Input: part model. Units: mm. Frame: model coordinates. Coordinates: 2 decimals unless noted, no trailing zeros. Order: outer loops, then holes, each group sorted by start corner. A loop starts at its lowest first (then second) coordinate and runs counter-clockwise, first axis right, second up. Notation, with made-up numbers: (17, 58) - (36, 58) arc R18 ccw to (36, 67) - close; hole circle Ø5 at (56.5, 79.25). An arc over 180 degrees is marked (long way). Answer as CSV lines item,"result". Start each with the question number.
Item 1: Material intervals for line 1 along X through (y, z) = (0.5, -184.5); line 2 along Y through (x, z) = (0, 91); line 3 along Y through (x, z) = (0, 218), sorted ascending.
Item 2: Section C-C (z = -195.5). Output: boundary loops of the cut face in (x, y), and give its area (3 significant figures).
Item 3: First-contact query: pin 1 (2 mm diameter, centred on y = -14, z = 18, fed in from -X); pin 2 (5 mm diameter, centred on y = 8, z = 146.5, fed in from -X); pin 3 (1.5 mm diameter, centred on y = 18.5, z = -55, fed in from -X). Flat tips, straight axial feed; report the tip coordinate or a pass-through.
Item 4: Section A-A (x = 0). Output: boundary loops of the cut face in (y, z).
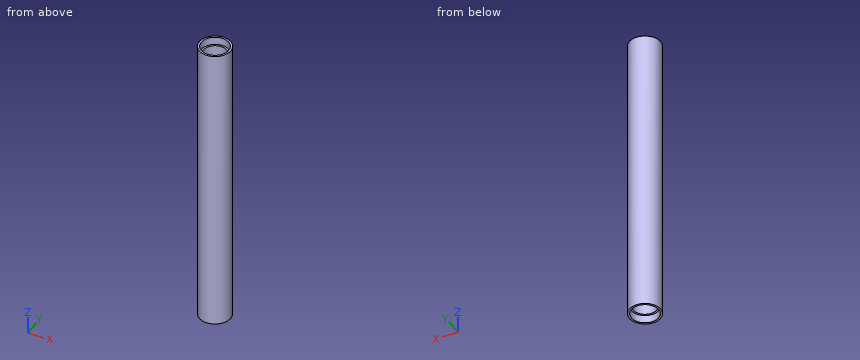
from build123d import *

# Parameters (mm, degrees)
SKETCH_1_R      = 24
SKETCH_1_R_2    = 21
EXTRUDE_1_DEPTH = 225
EXTRUDE_START   = -225
SKETCH_2_R      = 21
SKETCH_2_R_2    = 18
EXTRUDE_2_DEPTH = 213


with BuildPart() as part:
    # 草图1 → 拉伸-薄壁1 (new, symmetric)
    with BuildSketch(Plane.XY):
        Circle(SKETCH_1_R)
        Circle(SKETCH_1_R_2, mode=Mode.SUBTRACT)
    extrude(amount=EXTRUDE_1_DEPTH, both=True)

    # 草图2 → 拉伸-薄壁2 (add)
    with BuildSketch(Plane.XY.offset(225).offset(EXTRUDE_START)):
        Circle(SKETCH_2_R)
        Circle(SKETCH_2_R_2, mode=Mode.SUBTRACT)
    extrude_2 = extrude(amount=EXTRUDE_2_DEPTH)

    # 镜向1: 拉伸-薄壁2 across plane
    add(extrude_2.mirror(Plane.XY))


solid = part.part
Determined:
1,line 1,"x = -23.99 to -17.99, 17.99 to 23.99"
1,line 2,"y = -24 to -18, 18 to 24"
1,line 3,"y = -24 to -21, 21 to 24"
2,outline,"circle Ø48 at (0, 0); hole circle Ø36 at (0, 0)"
2,area,"792 mm^2"
3,pin 1,"stops at x = -20.17"
3,pin 2,"stops at x = -23.36"
3,pin 3,"stops at x = -16.15"
4,outline,"(-24, -225) - (-21, -225) - (-21, -213) - (-18, -213) - (-18, 213) - (-21, 213) - (-21, 225) - (-24, 225) - close; (18, -213) - (21, -213) - (21, -225) - (24, -225) - (24, 225) - (21, 225) - (21, 213) - (18, 213) - close"
